Input: dimensioned drawing with shaded views. Units: mm. Origin: part minimum x, y, z. Round coordinates to 2 decimals unless told otherwise and drop trailing zeros. Loops run counter-clockwise (first coordinate to the right, second up) from the corner with the lowest first, then second, coordinate; pieces in that order, holes last. Notation, with made-up numbers: M -32,88.25 L 16,88.25 A22 cw 16,94.25 Z; hole C 22.5,68 d2. An arc over 180 degrees is marked long. Return JSON: item names as keys, results as strings.
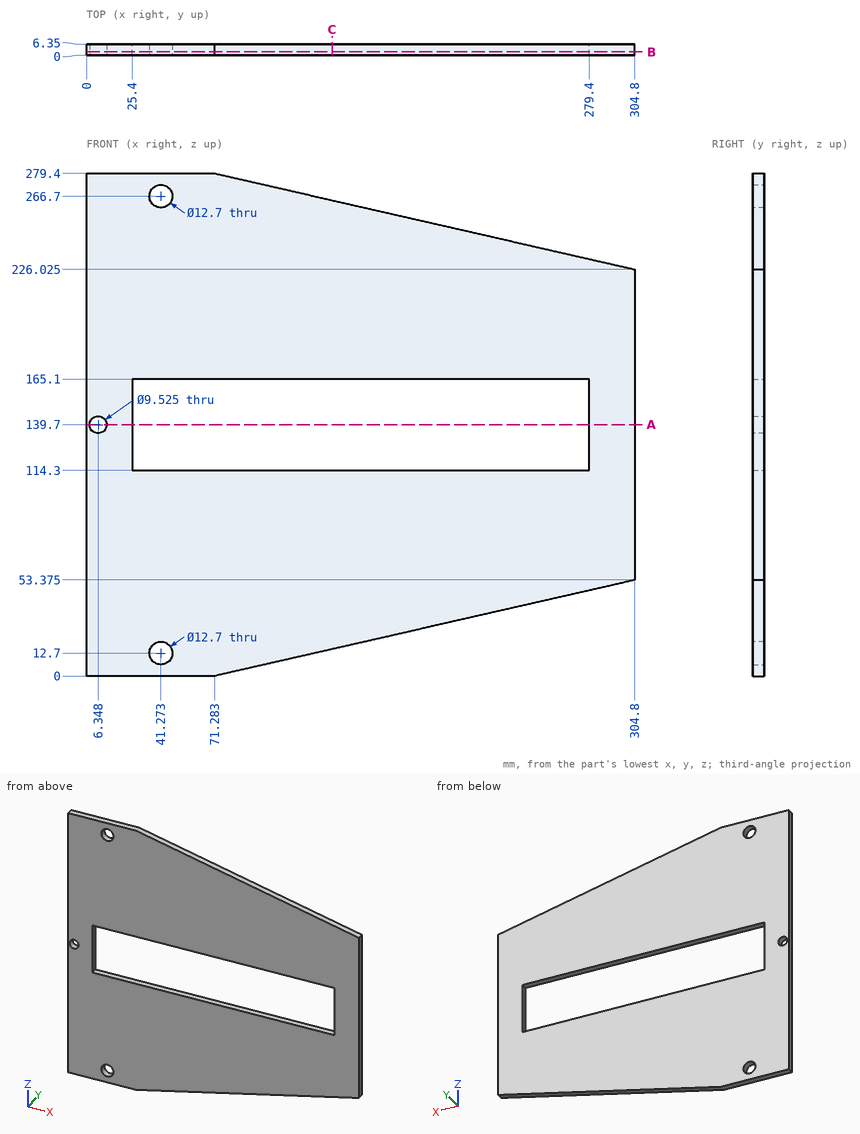
Q1. Section query B-B (y = 2). State how many separate pieces and enclosed holes the cut face has, plus the area to 3 significant figures.
Determined:
{"separate pieces": "1", "enclosed holes": "4", "area": "59,500 mm^2"}
Q2. Pin query (flat end, axial travel): pin 1 (1.9 mm diameter, centred on x = 209, y = 3.5, fed in from +Z); pin 2 (11.5 mm diameter, centred on x = 41.27, z = 266.7, fed in from -Y). Return the tip coordinate at first contact, or that it passes through.
Determined:
{"pin 1": "stops at z = 248.14", "pin 2": "passes through"}
Q3. Material intervals for L1, parallel to X at y = 2.25, z = 139.7; L2, parallel to Z at x = 27, y = 3.75; L3, parallel to Z at x = 214, y = 5.25, sorted ascending.
Determined:
{"L1": "x = 0 to 1.59, 11.11 to 25.4, 279.4 to 304.8", "L2": "z = 0 to 114.3, 165.1 to 279.4", "L3": "z = 32.62 to 114.3, 165.1 to 246.78"}
Q4. Section query C-C (x = 136.5). Output: boundary loops of the cut face in (y, z).
Determined:
{"outline": "M 0,14.91 L 6.35,14.91 L 6.35,114.3 L 0,114.3 Z; M 0,165.1 L 6.35,165.1 L 6.35,264.49 L 0,264.49 Z"}
Q5. Section query A-A (z = 139.7). Output: boundary loops of the cut face in (x, y), plus the area to 3 significant figures.
Determined:
{"outline": "M 0,0 L 1.59,0 L 1.59,6.35 L 0,6.35 Z; M 11.11,0 L 25.4,0 L 25.4,6.35 L 11.11,6.35 Z; M 279.4,0 L 304.8,0 L 304.8,6.35 L 279.4,6.35 Z", "area": "262 mm^2"}
